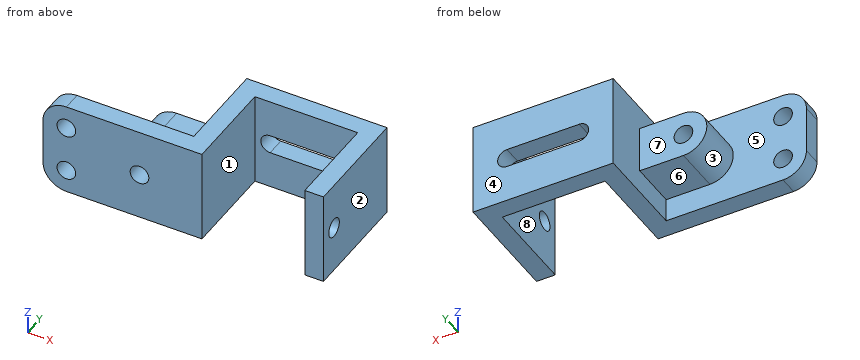
from build123d import *

# Parameters (mm, degrees)
BOSS_EXTRUDE1_DEPTH = 45
FILLET1_R           = 22.5
SKETCH2_R           = 9
CUT_EXTRUDE1_DEPTH  = 90
SKETCH3_R           = 9
BOSS_EXTRUDE2_DEPTH = 45
SKETCH4_R           = 9
CUT_EXTRUDE2_DEPTH  = 217.795410468
CUT_EXTRUDE3_DEPTH  = 45
SKETCH6_R           = 9
CUT_EXTRUDE4_DEPTH  = 45


with BuildPart() as part:
    # Sketch1 → Boss-Extrude1 (new, symmetric)
    with BuildSketch(Plane.XY):
        Polygon((-67.5, 108), (67.5, 108), (67.5, 0), (49.5, 0), (49.5, 90), (-49.5, 90), (-49.5, 0), (-67.5, 0), (-202.5, 0), (-202.5, 18), (-67.5, 18), align=None)
    extrude(amount=BOSS_EXTRUDE1_DEPTH, both=True)

    # Fillet1
    fillet1_edges = [part.edges().sort_by_distance(p)[0] for p in [
        (-202.5, 9, -45),
        (-202.5, 9, 45),
    ]]
    fillet(fillet1_edges, radius=FILLET1_R)

    # Sketch2 → Cut-Extrude1 (cut)
    with BuildSketch(Plane(origin=(0, 18, 0), x_dir=(1, 0, 0), z_dir=(0, 1, 0))):
        with Locations(Location((-180, -22.5, 0), (0, 0, 270))):
            Circle(SKETCH2_R)
        with Locations(Location((-180, 22.5, 0), (0, 0, 270))):
            Circle(SKETCH2_R)
    extrude(amount=-CUT_EXTRUDE1_DEPTH, mode=Mode.SUBTRACT)

    # Sketch3 → Boss-Extrude2 (add)
    with BuildSketch(Plane(origin=(0, 18, 0), x_dir=(1, 0, 0), z_dir=(0, 1, 0))):
        with BuildLine():
            Line((-67.5, 22.5), (-109.596739016, 22.5))
            ThreePointArc((-109.596739016, 22.5), (-132.096739016, 0), (-109.596739016, -22.5))
            Line((-109.596739016, -22.5), (-67.5, -22.5))
            Line((-67.5, -22.5), (-67.5, 22.5))
        make_face()
        with Locations(Location((-109.596739016, 0, 0), (0, 0, 90))):
            Circle(SKETCH3_R, mode=Mode.SUBTRACT)
    extrude(amount=BOSS_EXTRUDE2_DEPTH)

    # Sketch4 → Cut-Extrude2 (cut, through all)
    with BuildSketch(Plane(origin=(0, 63, 0), x_dir=(1, 0, 0), z_dir=(0, 1, 0))):
        with Locations(Location((-109.596739016, 0, 0), (0, 0, 90))):
            Circle(SKETCH4_R)
    extrude(amount=-CUT_EXTRUDE2_DEPTH, mode=Mode.SUBTRACT)

    # Sketch5 → Cut-Extrude3 (cut)
    with BuildSketch(Plane(origin=(0, 108, 0), x_dir=(1, 0, 0), z_dir=(0, 1, 0))):
        with BuildLine():
            Line((-34.803236343, 9), (34.803236343, 9))
            ThreePointArc((34.803236343, 9), (43.803236343, 0), (34.803236343, -9))
            Line((34.803236343, -9), (-34.803236343, -9))
            ThreePointArc((-34.803236343, -9), (-43.803236343, 0), (-34.803236343, 9))
        make_face()
    extrude(amount=-CUT_EXTRUDE3_DEPTH, mode=Mode.SUBTRACT)

    # Sketch6 → Cut-Extrude4 (cut)
    with BuildSketch(Plane(origin=(67.5, 0, 0), x_dir=(0, 0, -1), z_dir=(1, 0, 0))):
        with Locations((0, 18)):
            Circle(SKETCH6_R)
    extrude(amount=-CUT_EXTRUDE4_DEPTH, mode=Mode.SUBTRACT)


solid = part.part
Model file for the job. Use its own axes, mm. Face numbers are marked on the shaded views. A direction names the side the tool comes from. Coordinates: 2 decimals unless noted, no trailing zeros. Write each loop counter-clockwise with the first axis right and the second up, starting at its lowest first coordinate (ties: lowest second). Pieces come first, ordered by that corner, then holes. Notation, with made-up numbers: (71, -34.75) -> (99, -34.75) arc R26 cw to (99, -0.75) -> close; hole circle Ø9 at (41, -32). An arc over 180 degrees is marked (long way). One line per item, written item: value. Start each with the question number.
1) Pull direction X, two halves, no side cores. Call the marked faces 1, 2, 3 and 4: +X half, -X half, draft (parallel to the pull), parting line (faces both ways), or undercut.
2) Probe probe 1 along X at (y, z) = (13, -22); probe 2 along X at (y, z) = (83.5, 7); probe 3 along X at (y, z) = (51.5, -5.5). List the from-to ranges inside material, lowest first.
3) Slice it at B-B on z = 0. Write the cut outline in (x, y).
4) Slice it at C-C on y = 59.5. Write the cut outline in (x, z).
5) Which spindle directions (+Z, -Z, +X, -X, +Y, -Y) get a long thin tool onto all of the face, cutting with end or side? Do the marked faces 5, 6, 7 and 8. Say none if no direction does.
6) Slice it at D-D on y = 73. Write the cut outline in (x, z), then the cut area to 3 significant figures.
7) Flat gauge pins, fed straight in: pin 1 Ø1 at (x, y) = (-171, 20) entering from -Z; pin 2 Ø10 at (y, z) = (47.5, 29) entering from -X; pin 3 Ø3 at (x, z) = (-77.5, 5.5) entering from +Y; pin 4 Ø12.5 at (x, y) = (-89, 35.5) entering from -Z. Where does each tip first touch, or does it go through?
8) Slice it at A-A on x = 15. Write the cut outline in (y, z), then the cut area to 3 significant figures.
Answers follow:
1. face 1: undercut
1. face 2: +X half
1. face 3: -X half
1. face 4: draft
2. probe 1: -202.5 to -188.99, -171.01 to -49.5, 49.5 to 67.5
2. probe 2: -67.5 to -49.5, 49.5 to 67.5
2. probe 3: -131.41 to -116.72, -102.47 to -49.5, 49.5 to 67.5
3. outline: (-202.5, 0) -> (-118.6, 0) -> (-118.6, 63) -> (-132.1, 63) -> (-132.1, 18) -> (-202.5, 18) -> close; (-100.6, 0) -> (-49.5, 0) -> (-49.5, 90) -> (-43.8, 90) -> (-43.8, 108) -> (-67.5, 108) -> (-67.5, 63) -> (-100.6, 63) -> close; (43.8, 90) -> (49.5, 90) -> (49.5, 27) -> (67.5, 27) -> (67.5, 108) -> (43.8, 108) -> close; (49.5, 0) -> (67.5, 0) -> (67.5, 9) -> (49.5, 9) -> close
4. outline: (-109.6, -22.5) -> (-67.5, -22.5) -> (-67.5, -45) -> (-49.5, -45) -> (-49.5, 45) -> (-67.5, 45) -> (-67.5, 22.5) -> (-109.6, 22.5) arc R22.5 ccw to start; (49.5, -45) -> (67.5, -45) -> (67.5, 45) -> (49.5, 45) -> close; hole circle Ø18 at (-109.6, 0)
5. face 5: -X, +Y
5. face 6: -Z, -X, +Y
5. face 7: +Z, -Z, -X, +Y
5. face 8: +Z, -Z, -Y
6. outline: (-67.5, -45) -> (-49.5, -45) -> (-49.5, 45) -> (-67.5, 45) -> close; (49.5, -45) -> (67.5, -45) -> (67.5, 45) -> (49.5, 45) -> close
6. area: 3,240 mm2
7. pin 1: through
7. pin 2: x = -67.5
7. pin 3: y = 63
7. pin 4: z = -22.5
8. outline: (90, -45) -> (108, -45) -> (108, -9) -> (90, -9) -> close; (90, 9) -> (108, 9) -> (108, 45) -> (90, 45) -> close
8. area: 1,300 mm2
